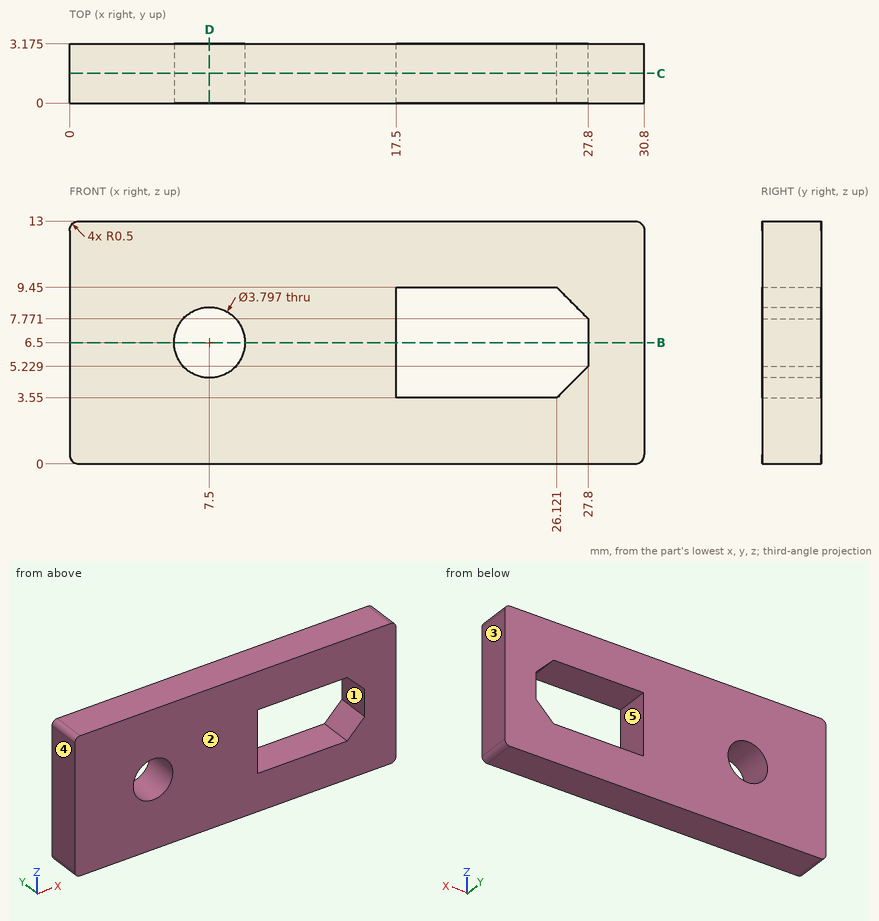
Input: dimensioned drawing with shaded views. Units: mm. Origin: part minimum x, y, z. A direction names the side the tool comes from. Coordinates: 2 decimals unless noted, no trailing zeros. Order: outer loops, then holes, each group sorted by start corner. A loop starts at its lowest first (then second) coordinate and runs counter-clockwise, first axis right, second up.
(1) Section query B-B (z = 6.5). Return the cut outline in (x, y) (1 decimal).
(2) Material intervals for probe 1 along X at (y, z) = (1.3, 6.5); probe 2 along Z at (x, y) = (19, 2.3); probe 3 along X at (y, z) = (1.45, 7.75), sorted ascending.
(3) Section query D-D (x = 7.5). Return the cut outline in (y, z) (1 decimal), plus the area to 3 significant figures.
(4) Access query for the marked faces 1 and 2. Directions: +Z, -Z, +X, -X, +Y, -Y. A direction counts if a zero-diameter tool reaches every point of the face in a straight line with its end or side. Return the directions, or none.
(5) Section query C-C (y = 1.6). Return the cut outline in (x, z), plus the area to 3 significant figures.
(6) Draft query along X for the marked faces 3, 4 and 5. Return one class per face: pulls with the +X half, pulls with the -X half, needs draft (parallel to the pull), parting line crosses it, or undercut.
(7) First-contact query: pin 1 (1 mm diameter, centred on x = 23, y = 1, fed in from -Z); pin 2 (3 mm diameter, centred on x = 7.5, z = 6.5, fed in from +Y). Flat tips, straight axial feed; report the tip coordinate or a pass-through.
Solution:
1. outline: (0, 0) - (5.6, 0) - (5.6, 3.2) - (0, 3.2) - close; (9.4, 0) - (17.5, 0) - (17.5, 3.2) - (9.4, 3.2) - close; (27.8, 0) - (30.8, 0) - (30.8, 3.2) - (27.8, 3.2) - close
2. probe 1: x = 0 to 5.6, 9.4 to 17.5, 27.8 to 30.8
2. probe 2: z = 0 to 3.55, 9.45 to 13
2. probe 3: x = 0 to 6.07, 8.93 to 17.5, 27.8 to 30.8
3. outline: (0, 0) - (3.2, 0) - (3.2, 4.6) - (0, 4.6) - close; (0, 8.4) - (3.2, 8.4) - (3.2, 13) - (0, 13) - close
3. area: 29.2 mm2
4. face 1: +Y, -Y
4. face 2: +Z, -Z, +X, -X, -Y
5. outline: (0, 0.5) arc R0.5 ccw to (0.5, 0) - (30.3, 0) arc R0.5 ccw to (30.8, 0.5) - (30.8, 12.5) arc R0.5 ccw to (30.3, 13) - (0.5, 13) arc R0.5 ccw to (0, 12.5) - close; hole circle Ø3.8 at (7.5, 6.5); hole (17.5, 3.55) - (26.12, 3.55) - (27.8, 5.23) - (27.8, 7.77) - (26.12, 9.45) - (17.5, 9.45) - close
5. area: 331 mm2
6. face 3: pulls with the +X half
6. face 4: pulls with the -X half
6. face 5: undercut
7. pin 1: stops at z = 0
7. pin 2: passes through
